Geometry check sheet. Reference: the model listing, model coordinates, mm. Round coordinates to 2 decimals unless told otherwise and drop trailing zeros. Order: outer loops, then holes, each group sorted by start corner. A loop starts at its lowest first (then second) coordinate and runs counter-clockwise, first axis right, second up. Notation, with made-up numbers: (65, -10) - (86, -10) arc R18 cw to (86, -1) - close; hole circle Ø2 at (69.25, 34.5). An arc over 180 degrees is marked (long way). Use a Markdown table: item, result. Add a question column.
(1) Gauge pin test, flat ends, axial feed: P1, Ø2, axis at x = 1.5, z = -16.5, coming from the -Y side; P2, Ø2, axis at x = 1.5, z = -18, coming from the -Y side; P3, Ø5, axis at x = -3.5, z = -5.5, coming from the +Y side. Record the tip position at first contact, or that the pin passes through.
(2) Thickness scan on line 1 along X through (y, z) = (-115, -5.25); line 2 along Y through (x, z) = (-5.75, -11.5); line 3 along Y through (x, z) = (-0.5, -8.5). Record the ranges inside material, lowest first. Write a range as [from, to].
(3) Section check C-C on z = -18.75. Record the boundary of the cut face in (x, y), then the cut area to 3 significant figures.
(4) Mould release check, pull along Y, two halves, no side actions. Record for faces 1 (the face through (0, -150, -10)), 2 (the face through (0, -3, 0)), 3 (the face through (0.11, -170.72, -20.49)): released by +Y, released by -Y, zero draft, split by the parting line, or undercut.
(5) Section check B-B on x = -3.5. Record the boundary of the cut face in (y, z).
(6) Section check A-A on y = 135. Record the boundary of the cut face in (x, z), then the cut area to 3 significant figures.
```python
from build123d import *

# Parameters (mm, degrees)
F0_R     = 5
F1_DEPTH = 8
F2_R     = 1
F3_DEPTH = 25.001


with BuildPart() as f1:
    # F0 (on Right) → F1 (new body, symmetric)
    with BuildSketch(Plane.YZ):
        with BuildLine():
            ThreePointArc((175, -10), (172.071068, -2.928932), (165, 0))
            Line((165, 0), (-175, 0))
            Line((-175, 0), (-175, -10))
            ThreePointArc((-175, -10), (-170.606602, -20.606602), (-160, -25))
            Line((-160, -25), (160, -25))
            ThreePointArc((160, -25), (170.606602, -20.606602), (175, -10))
        make_face()
        with Locations((-145, -10)):
            Circle(F0_R, mode=Mode.SUBTRACT)
        with Locations((135, -10)):
            Circle(F0_R, mode=Mode.SUBTRACT)
    extrude(amount=F1_DEPTH, both=True)

    # F2 (on Top) → F3 (cut, through all)
    with BuildSketch(Plane.XY):
        with Locations((0, 65)):
            Circle(F2_R)
        with Locations((0, -115)):
            Circle(F2_R)
    extrude(amount=-F3_DEPTH, mode=Mode.SUBTRACT)


solid = f1.part
```
Check sheet entries:
| question | item | result |
|---|---|---|
| 1 | P1 | stops at y = -173.96 |
| 1 | P2 | stops at y = -173.27 |
| 1 | P3 | stops at y = 174.8 |
| 2 | line 1 | x = [-8, -1], [1, 8] |
| 2 | line 2 | y = [-174.92, -149.77], [-140.23, 130.23], [139.77, 174.92] |
| 2 | line 3 | y = [-175, -149.77], [-140.23, -115.87], [-114.13, 64.13], [65.87, 130.23], [139.77, 174.89] |
| 3 | outline | (-8, -172.18) - (8, -172.18) - (8, 172.18) - (-8, 172.18) - close; hole circle Ø2 at (0, -115); hole circle Ø2 at (0, 65) |
| 3 | area | 5,500 mm2 |
| 4 | face 1 | undercut |
| 4 | face 2 | zero draft |
| 4 | face 3 | released by -Y |
| 5 | outline | (-175, -10) arc R15 ccw to (-160, -25) - (160, -25) arc R15 ccw to (175, -10) arc R10 ccw to (165, 0) - (-175, 0) - close; hole circle Ø10 at (-145, -10); hole circle Ø10 at (135, -10) |
| 6 | outline | (-8, -25) - (8, -25) - (8, -15) - (-8, -15) - close; (-8, -5) - (8, -5) - (8, 0) - (-8, 0) - close |
| 6 | area | 240 mm2 |
